Model file for the job. Use its own axes, mm. A direction names the side the tool comes from. Give positions to 0.01 mm unless a question says otherwise; leave off trailing zeros. Loops run counter-clockwise (first coordinate to the right, second up) from the corner with the lowest first, then second, coordinate; pieces in that order, holes last. Notation, with made-up numbers: (47.5, 47) - (87.5, 47) arc R19 ccw to (87.5, 54) - close; hole circle Ø10 at (-26.75, 28.25). An arc over 180 degrees is marked (long way). Answer as CSV lines item,"result". Start each with the question number.
Item 1: Drill centre lines: L1, parallel to Y at x = 0, z = 134.5; L2, parallel to X at y = 16, z = 144; L3, parallel to X at y = -40, z = 97. Where is each one in solid material? Low to high. Write a range as from..to.
Item 2: Tool access for faces 4 (the flat face through (0, 0, 191)), 5 (the flat face through (0, -40, 130)): list every direction of +Z, -Z, +X, -X, +Y, -Y with a clear straight run to the whole face (end or side of a thin tool).
Item 3: Saw through at A-A on y = 0. Give the cut face in (x, z), plus the area to 3 significant figures.
Item 4: Pin check, flat tips, straight feed: pin 1 (2 mm diameter, centred on x = -13.5, y = -38.5, fed in from -Z); pin 2 (12 mm diameter, centred on x = 4.5, z = 28.5, fed in from +Y); pin 3 (7.5 mm diameter, centred on x = -30, y = -16.5, fed in from +Z); pin 4 (17 mm diameter, centred on x = 33.04, y = 19.07, fed in from +Z). Stop position of each tip, or through.
Item 5: Saw through at B-B on x = 0. Give the cut face in (y, z), plus the area to 3 significant figures.
Item 6: Saw through at D-D on y = -14.5. Give the cut face in (x, z).
Item 7: Pull direction X, two halves, no side cores. Call faces 1 (the flat face through (6, -20, 156)), 2 (the cylindrical face through (-3.921, -45.724, 140.14)), 3 (the cylindrical face through (-2.17, -9.76, 175.79)): pulls with the +X half, pulls with the -X half, needs draft (parallel to the pull), parting line crosses it, or undercut.
Item 8: Saw through at C-C on z = 106. Give the cut face in (x, y), plus the area to 3 significant figures.
from build123d import *

# Parameters (mm, degrees)
SKETCH_4_R          = 50
EXTRUDE_1_DEPTH     = 150
SKETCH_5_R          = 30
EXTRUDE_2_DEPTH     = 6
SKETCH_6_R          = 20
EXTRUDE_3_DEPTH     = 5
SKETCH_7_R          = 10
EXTRUDE_4_DEPTH     = 30
SKETCH_8_R          = 7.293017107
CUT_EXTRUDE_1_DEPTH = 20


with BuildPart() as part:
    # 草图4 → 凸台-拉伸1 (new body)
    with BuildSketch(Plane.XY):
        Circle(SKETCH_4_R)
    extrude(amount=EXTRUDE_1_DEPTH)

    # 草图5 → 凸台-拉伸2 (add)
    with BuildSketch(Plane.XY.offset(150)):
        Circle(SKETCH_5_R)
    extrude(amount=EXTRUDE_2_DEPTH)

    # 草图6 → 凸台-拉伸3 (add)
    with BuildSketch(Plane.XY.offset(156)):
        Circle(SKETCH_6_R)
    extrude(amount=EXTRUDE_3_DEPTH)

    # 草图7 → 凸台-拉伸4 (add)
    with BuildSketch(Plane.XY.offset(161)):
        Circle(SKETCH_7_R)
    extrude(amount=EXTRUDE_4_DEPTH)

    # 草图8 → 切除-拉伸1 (cut)
    with BuildSketch(Plane.XY.offset(150)):
        with Locations((0, 39.574124617)):
            Circle(SKETCH_8_R)
        with Locations((33.03726858, 19.074075908)):
            Circle(SKETCH_8_R)
        with Locations(Location((0, -39.574124617, 0), (0, 0, 180))):
            Circle(SKETCH_8_R)
        with Locations(Location((-33.03726858, 19.074075908, 0), (0, 0, 180))):
            Circle(SKETCH_8_R)
        with Locations(Location((33.03726858, -19.074075908, 0), (0, 0, 180))):
            Circle(SKETCH_8_R)
        with Locations((-33.03726858, -19.074075908)):
            Circle(SKETCH_8_R)
    extrude(amount=-CUT_EXTRUDE_1_DEPTH, mode=Mode.SUBTRACT)


solid = part.part
Responses:
1,L1,"-50..-46.87, -32.28..32.28, 46.87..50"
1,L2,"-47.37..-39.65, -26.42..26.42, 39.65..47.37"
1,L3,"-30..30"
2,face 4,"+Z, +X, -X, +Y, -Y"
2,face 5,"+Z"
3,outline,"(-50, 0) - (50, 0) - (50, 150) - (30, 150) - (30, 156) - (20, 156) - (20, 161) - (10, 161) - (10, 191) - (-10, 191) - (-10, 161) - (-20, 161) - (-20, 156) - (-30, 156) - (-30, 150) - (-50, 150) - close"
3,area,"16,200 mm2"
4,pin 1,"z = 0"
4,pin 2,"y = 50"
4,pin 3,"z = 150"
4,pin 4,"z = 156"
5,outline,"(-50, 0) - (50, 0) - (50, 150) - (46.87, 150) - (46.87, 130) - (32.28, 130) - (32.28, 150) - (30, 150) - (30, 156) - (20, 156) - (20, 161) - (10, 161) - (10, 191) - (-10, 191) - (-10, 161) - (-20, 161) - (-20, 156) - (-30, 156) - (-30, 150) - (-32.28, 150) - (-32.28, 130) - (-46.87, 130) - (-46.87, 150) - (-50, 150) - close"
5,area,"15,600 mm2"
6,outline,"(-47.85, 0) - (47.85, 0) - (47.85, 150) - (38.72, 150) - (38.72, 130) - (27.36, 130) - (27.36, 150) - (26.26, 150) - (26.26, 156) - (13.77, 156) - (13.77, 161) - (-13.77, 161) - (-13.77, 156) - (-26.26, 156) - (-26.26, 150) - (-27.36, 150) - (-27.36, 130) - (-38.72, 130) - (-38.72, 150) - (-47.85, 150) - close"
7,face 1,"needs draft"
7,face 2,"undercut"
7,face 3,"parting line crosses it"
8,outline,"circle Ø100 at (0, 0)"
8,area,"7,850 mm2"
